Solid Edge part; units mm, degrees
sketch "Sketch1" plane through (0, 0, 0) normal (0, 0, 1) x (1, 0, 0)
  line L0 (100, -100) -> (100, 100)
  line L1 (100, 100) -> (-100, 100)
  line L2 (-100, 100) -> (-100, -100)
  line L3 (-100, -100) -> (100, -100)
extrude "Protrusion1" add sketch "Sketch1" along normal blind 230
sketch "Sketch2" plane through (0, 0, 0) normal (0, 0, -1) x (0, 1, 0)
  line L0 (-90, 90) -> (-90, -90)
  line L1 (-90, -90) -> (90, -90)
  line L2 (90, -90) -> (90, 90)
  line L3 (90, 90) -> (-90, 90)
extrude "ScavoEstrusione_1" cut sketch "Sketch2" against normal blind 210
sketch "Sketch3" plane through (-100, 0, 114.7797) normal (-1, 0, 0) x (0, -1, 0)
  line L0 (-90, 95.1431) -> (90, 95.1431)
  line L1 (90, 95.1431) -> (90, -39.2912)
  line L2 (90, -39.2912) -> (-90, -39.2912)
  line L3 (-90, -39.2912) -> (-90, 95.1431)
extrude "ScavoEstrusione_2" cut sketch "Sketch3" against normal blind 30
sketch "Sketch4" plane through (0, -100, 115) normal (0, -1, 0) x (1, 0, 0)
  line L0 (-34.2156, 73.853) -> (-34.2156, -95.3257)
  line L1 (-34.2156, -105.591) -> (-34.2156, -95.3257)
  line L2 (-89.2156, -105.591) -> (-34.2156, -105.591)
  line L3 (-89.2156, -95.3257) -> (-89.2156, -105.591)
  line L4 (-89.2156, -95.3257) -> (-89.2156, 73.853)
  line L5 (-89.2156, 73.853) -> (-89.2156, 91.853)
  line L6 (-89.2156, 91.853) -> (-34.2156, 91.853)
  line L7 (-34.2156, 91.853) -> (-34.2156, 73.853)
  line L8 (32.7844, -105.591) -> (32.7844, 91.853)
  line L9 (-30.2156, 91.853) -> (32.7844, 91.853)
  line L10 (-30.2156, 73.853) -> (-30.2156, 91.853)
  line L11 (-30.2156, -105.591) -> (-30.2156, 73.853)
  line L12 (19.3173, -105.591) -> (-30.2156, -105.591)
  line L13 (32.7844, -105.591) -> (19.3173, -105.591)
  line L14 (36.7844, 91.853) -> (96.7844, 91.853)
  line L15 (96.7844, 91.853) -> (96.7844, 73.853)
  line L16 (96.7844, 73.853) -> (96.7844, -105.591)
  line L17 (96.7844, -105.591) -> (36.7844, -105.591)
  line L18 (36.7844, 91.853) -> (36.7844, -105.591)
extrude "ScavoEstrusione_3" cut sketch "Sketch4" against normal blind 317.7816
sketch "Sketch5" plane through (100, 0, 115) normal (1, 0, 0) x (0, 1, 0)
  line L0 (-90, 73.853) -> (-35, 73.853)
  line L1 (-35, 73.853) -> (-35, -95.3257)
  line L2 (-35, -95.3257) -> (-90, -95.3257)
  line L3 (-90, -95.3257) -> (-90, 73.853)
  line L4 (-31, 91.853) -> (32, 91.853)
  line L5 (32, -105.591) -> (32, 91.853)
  line L6 (32, -105.591) -> (18.5329, -105.591)
  line L7 (18.5329, -105.591) -> (-31, -105.591)
  line L8 (-31, -105.591) -> (-31, 73.853)
  line L9 (-31, 73.853) -> (-31, 91.853)
  line L10 (36, 91.853) -> (36, -105.591)
  line L11 (96, -105.591) -> (36, -105.591)
  line L12 (96, 73.853) -> (96, -105.591)
  line L13 (96, 91.853) -> (96, 73.853)
  line L14 (36, 91.853) -> (96, 91.853)
extrude "ProtrusioneEstrusa_3" cut sketch "Sketch5" against normal blind 166.3749
Design review of the part built by this model. Coordinates are the model's own, in mm. A direction names the side the tool comes from. Round coordinates to 2 decimals unless told otherwise and drop trailing zeros. Write each loop counter-clockwise with the first axis right and the second up, starting at its lowest first coordinate (ties: lowest second). Pieces come first, ordered by that corner, then holes. Notation, with made-up numbers: (-4.5, 66) - (34.5, 66) arc R34 cw to (34.5, 96) - close; hole circle Ø11 at (4.5, -1.75). An arc over 180 degrees is marked (long way). Return JSON: item names as keys, results as strings. Group by question number.
Item 1: We need section C-C on z = 200.5. Give the number of separate pieces and of enclosed holes in the cut face, and give its area (3 significant figures).
Item 2: For probe 1 along Z at (x, y) = (-75, -76.5); probe 2 along X at (y, z) = (-53, 28); probe 3 along Y at (x, z) = (35.5, 60.5), list the stretches that pass through material, from the lowest coordinate up. Write a range as [from, to].
Item 3: The part is to be moulded in two halves that separate along X. For faces 1 (the face through (-8, -96, 0)), 2 (the face through (90, 1, 5)), 3 (the face through (-100, 1, 62)), say which applies: pulls with the +X half, pulls with the -X half, needs draft (parallel to the pull), parting line crosses it, or undercut.
Item 4: We need section D-D on y = -5. Write out the cut boundary in (x, z).
Item 5: We need section B-B on x = -20. Write out the cut boundary in (y, z), and give its area (3 significant figures).
Item 6: Insertion check: P1, Ø10, axis at x = 38.5, z = 123.5, coming from the -Y side; P2, Ø12, axis at x = -69, y = 44.5, coming from the -Z side. Each pin has a flat end and moves straight along its axis. Give the tip position at first contact, or say it passes through.
Item 7: We need section A-A on y = -78.5. Write out the cut boundary in (x, z).
Item 8: Machinability: for faces 4 (the face through (-95, 1, 209.923)), 5 (the face through (-30.216, -95, 107)), 6 (the face through (97, 45, 9.409)), 7 (the face through (36.6, -100, 140)), which of the approach directions +Z, -Z, +X, -X, +Y, -Y give a long, thin tool a straight path to every point of the face, cutting with its end or side? Answer none if there is none.
Model answer:
{
 "1": {"separate pieces": "9", "enclosed holes": "0", "area": "575 mm²"},
 "2": {"probe 1": "z = [210, 230]", "probe 2": "x = [-100, -90]", "probe 3": "y = [-100, -90], [96, 100]"},
 "3": {"face 1": "needs draft", "face 2": "undercut", "face 3": "pulls with the -X half"},
 "4": {"outline": "(-100, 0) - (-90, 0) - (-90, 75.49) - (-100, 75.49) - close; (-100, 209.92) - (-90, 209.92) - (-90, 210) - (90, 210) - (90, 206.85) - (100, 206.85) - (100, 230) - (-100, 230) - close; (90, 0) - (100, 0) - (100, 9.41) - (90, 9.41) - close"},
 "5": {"outline": "(-100, 0) - (-90, 0) - (-90, 9.41) - (-100, 9.41) - close; (-100, 206.85) - (-90, 206.85) - (-90, 210) - (90, 210) - (90, 206.85) - (100, 206.85) - (100, 230) - (-100, 230) - close; (90, 0) - (100, 0) - (100, 9.41) - (90, 9.41) - close", "area": "4,250 mm²"},
 "6": {"P1": "stops at y = -100", "P2": "stops at z = 210"},
 "7": {"outline": "(-100, 0) - (-90, 0) - (-90, 75.49) - (-100, 75.49) - close; (-100, 209.92) - (-90, 209.92) - (-90, 210) - (90, 210) - (90, 206.85) - (96.78, 206.85) - (96.78, 188.85) - (100, 188.85) - (100, 230) - (-100, 230) - close; (90, 0) - (100, 0) - (100, 19.67) - (96.78, 19.67) - (96.78, 9.41) - (90, 9.41) - close"},
 "8": {"face 4": "-X", "face 5": "+Y, -Y", "face 6": "none", "face 7": "+Z, -Z, +X, -X, -Y"}
}
